Input: dimensioned drawing with shaded views. Units: mm. Origin: part minimum x, y, z. Coordinates: 2 decimals unless noted, no trailing zeros. Order: outer loops, then holes, each group sorted by start corner. A loop starts at its lowest first (then second) coordinate and runs counter-clockwise, first axis right, second up. Notation, with made-up numbers: (-17.75, 18.25) -> (17.25, 18.25) arc R24 cw to (17.25, 53.25) -> close; hole circle Ø11 at (49.5, -36). An arc over 180 degrees is marked (long way). Put each result on its own line as item: value.
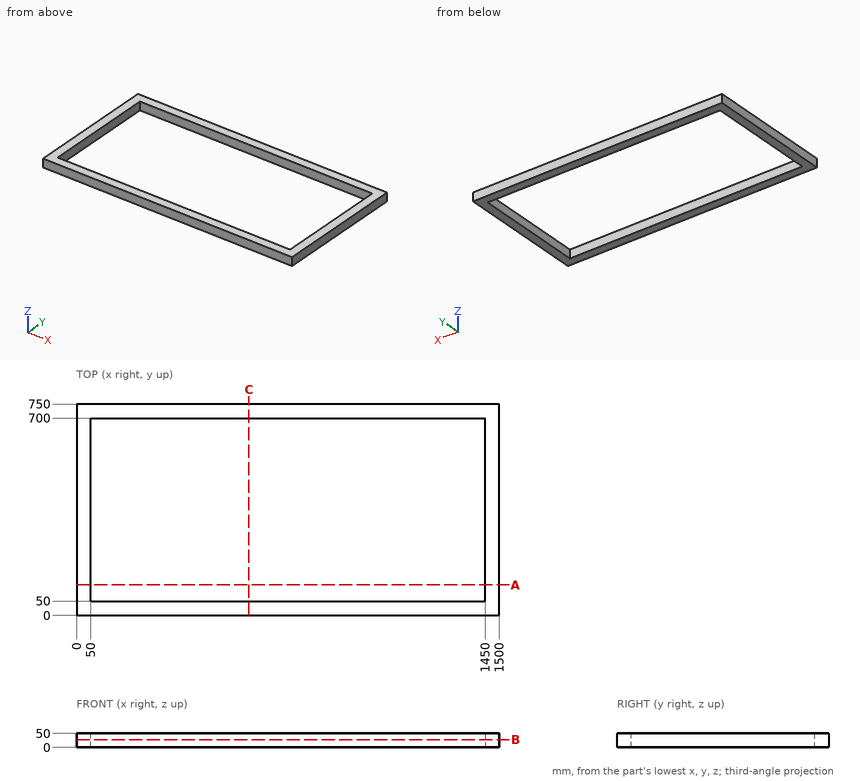
1. Cut plane A-A on y = 108. Output: boundary loops of the cut face in (x, z), plus the area to 3 significant figures.
Numbers:
outline: (0, 0) -> (50, 0) -> (50, 50) -> (0, 50) -> close; (1450, 0) -> (1500, 0) -> (1500, 50) -> (1450, 50) -> close
area: 5,000 mm2
2. Cut plane C-C on x = 611.5. Output: boundary loops of the cut face in (y, z), plus the area to 3 significant figures.
Numbers:
outline: (0, 0) -> (50, 0) -> (50, 50) -> (0, 50) -> close; (700, 0) -> (750, 0) -> (750, 50) -> (700, 50) -> close
area: 5,000 mm2
3. First-contact query: pin 1 (15 mm diameter, centred on x = 577, z = 23, fed in from -Y). Flat tip, straight axial feed; report the tip coordinate or a pass-through.
Numbers:
pin 1: stops at y = 0
4. Ray query, line 1 along X through (y, z) = (327, 48); line 2 along Y through (x, z) = (756, 46). Return the intervals inside material, ascending.
Numbers:
line 1: x = 0 to 50, 1450 to 1500
line 2: y = 0 to 50, 700 to 750
5. Cut plane B-B on z = 28. Output: boundary loops of the cut face in (x, y).
Numbers:
outline: (0, 0) -> (1500, 0) -> (1500, 750) -> (0, 750) -> close; hole (50, 50) -> (1450, 50) -> (1450, 700) -> (50, 700) -> close
